Source: CAD feature listing. Evaluate the final solid. Frame: model axes, mm. Face numbers are marked on the shaded views. Round coordinates to 2 decimals unless told otherwise and drop trailing zeros. Loops run counter-clockwise (first coordinate to the right, second up) from the corner with the lowest first, then second, coordinate; pieces in that order, holes last. Notation, with made-up numbers: M -28.75,51 L 27.25,51 A20 cw 27.25,65 Z; hole C 5.25,63.25 d8. An arc over 180 degrees is marked long. One line per item, written item: value.
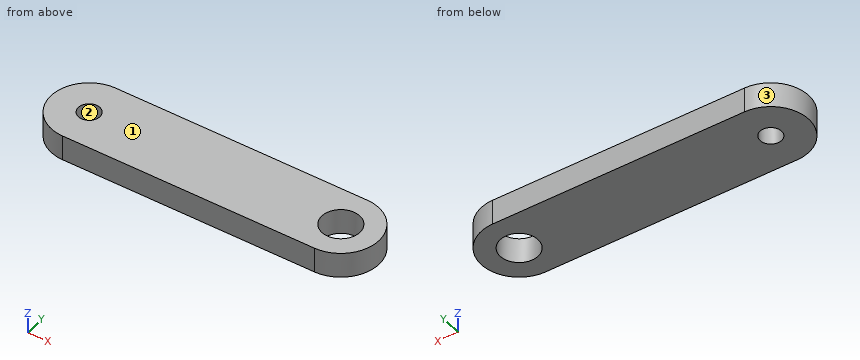
from build123d import *

# Parameters (mm, degrees)
SKETCH_1_R      = 1.5
EXTRUDE_1_DEPTH = 2
SKETCH_4_R      = 1.5
SKETCH_4_R_2    = 0.85
EXTRUDE_6_DEPTH = 2


with BuildPart() as part:
    # 草图1 → 凸台-拉伸1 (new body)
    with BuildSketch(Plane.XY):
        with BuildLine():
            Line((0, 3), (20, 3))
            ThreePointArc((20, 3), (23, 0), (20, -3))
            Line((20, -3), (0, -3))
            ThreePointArc((0, -3), (-3, 0), (0, 3))
        make_face()
        Circle(SKETCH_1_R, mode=Mode.SUBTRACT)
        with Locations((20, 0)):
            Circle(SKETCH_1_R, mode=Mode.SUBTRACT)
    extrude(amount=EXTRUDE_1_DEPTH)

    # 草图4 → 凸台-拉伸6 (add, through all)
    with BuildSketch(Plane(origin=(0, 0, 0), x_dir=(-1, 0, 0), z_dir=(0, 0, -1))):
        Circle(SKETCH_4_R)
        Circle(SKETCH_4_R_2, mode=Mode.SUBTRACT)
    extrude(amount=-EXTRUDE_6_DEPTH)


solid = part.part
1. Section query D-D (y = 2.6). Return the cut outline in (x, z), and give its area (3 significant figures).
Report:
outline: M -1.5,0 L 21.5,0 L 21.5,2 L -1.5,2 Z
area: 46.0 mm2
2. Section query A-A (y = 0). Return the cut outline in (x, z), and give its area (3 significant figures).
Report:
outline: M -3,0 L -0.85,0 L -0.85,2 L -3,2 Z; M 0.85,0 L 18.5,0 L 18.5,2 L 0.85,2 Z; M 21.5,0 L 23,0 L 23,2 L 21.5,2 Z
area: 42.6 mm2
3. Pull-direction query (X, two-part tool) for the marked faces 1, 2 and 3; classes: released by +X, released by -X, zero draft, split by the parting line, or undercut.
Report:
face 1: zero draft
face 2: undercut
face 3: released by -X
4. Section query C-C (x = 19.25). Return the cut outline in (y, z), and give its area (3 significant figures).
Report:
outline: M -3,0 L -1.3,0 L -1.3,2 L -3,2 Z; M 1.3,0 L 3,0 L 3,2 L 1.3,2 Z
area: 6.80 mm2
5. Pin query (flat end, axial travel): pin 1 (1.5 mm diameter, centred on x = 0, y = 0, fed in from +Z); pin 2 (1 mm diameter, centred on y = -2.5, z = 0.5, fed in from -X); pin 3 (3 mm diameter, centred on x = 9.5, y = -1, fed in from -Z). Return the tip coordinate at first contact, or that it passes through.
Report:
pin 1: passes through
pin 2: stops at x = -2.24
pin 3: stops at z = 0
6. Ray query, line 1 (Y direction, x = 0, z = 0.8); line 2 (Y direction, x = 20, z = 1.4); line 3 (X direction, y = 0.3, z = 1.8). Return the intervals inside material, ascending. Write a range as [from, to].
Report:
line 1: y = [-3, -0.85], [0.85, 3]
line 2: y = [-3, -1.5], [1.5, 3]
line 3: x = [-2.98, -0.8], [0.8, 18.53], [21.47, 22.98]
7. Section query B-B (z = 0.65). Return the cut outline in (x, y).
Report:
outline: M 0,-3 L 20,-3 A3 ccw 20,3 L 0,3 A3 ccw Z; hole C 0,0 d1.7; hole C 20,0 d3
